Geometry check sheet. Reference: the model listing, model coordinates, mm. Face numbers are marked on the shaded views. A direction names the side the tool comes from. Coordinates: 2 decimals unless noted, no trailing zeros. Loops run counter-clockwise (first coordinate to the right, second up) from the corner with the lowest first, then second, coordinate; pieces in that order, holes last. Notation, with made-up numbers: (82.5, 26.25) -> (120.5, 26.25) arc R11 ccw to (120.5, 37.25) -> close; hole circle Ø3 at (45.5, 13). An arc over 180 degrees is marked (long way). Answer as a JSON object with one key per item and string values.
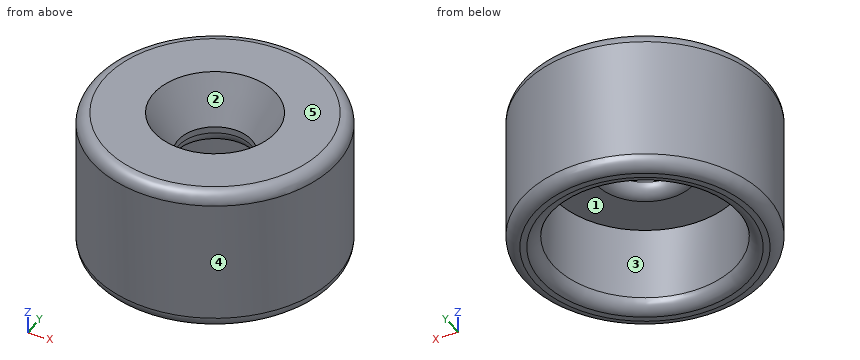
from build123d import *

# Parameters (mm, degrees)
SKETCH1_R           = 5
SKETCH1_R_2         = 1.5
BOSS_EXTRUDE1_DEPTH = 6
SKETCH2_R           = 3.75
CUT_EXTRUDE1_DEPTH  = 3.5
FILLET1_R           = 0.5
CHAMFER1_SIZE       = 1
CHAMFER1_SIZE2      = 1.732050808


with BuildPart() as part:
    # Sketch1 → Boss-Extrude1 (new body)
    with BuildSketch(Plane.XY):
        Circle(SKETCH1_R)
        Circle(SKETCH1_R_2, mode=Mode.SUBTRACT)
    extrude(amount=BOSS_EXTRUDE1_DEPTH)

    # Sketch2 → Cut-Extrude1 (cut)
    with BuildSketch(Plane.XY):
        Circle(SKETCH2_R)
    extrude(amount=CUT_EXTRUDE1_DEPTH, mode=Mode.SUBTRACT)

    # Fillet1
    fillet1_edges = [part.edges().sort_by_distance(p)[0] for p in [
        (-1.5, 0, 3.5),
        (-3.75, 0, 0),
        (-5, 0, 0),
        (-5, 0, 6),
    ]]
    fillet(fillet1_edges, radius=FILLET1_R)

    # Chamfer1
    chamfer1_edges = [part.edges().sort_by_distance(p)[0] for p in [
        (-1.5, 0, 6),
    ]]
    chamfer1_side = [part.faces().sort_by_distance(p)[0] for p in [
        (-4.372720779, 0, 6),
    ]]
    chamfer(chamfer1_edges, length=CHAMFER1_SIZE, length2=CHAMFER1_SIZE2, reference=chamfer1_side[0])


solid = part.part
1. Tool access check on the marked faces 1 and 2. Record the directions out of +Z, -Z, +X, -X, +Y, -Y that give a thin tool (end or side, any length) a straight path to the whole face; none if there is none.
Evaluation:
{"face 1": "-Z", "face 2": "+Z"}
2. Section check D-D, the plane z = 5.1. Record the boundary of the cut face in (x, y).
Evaluation:
{"outline": "circle Ø10 at (0, 0); hole circle Ø3.96 at (0, 0)"}
3. Thickness scan on probe 1 along Y at (x, z) = (0, 2.8); probe 2 along Y at (x, z) = (0, 4.1); probe 3 along X at (y, z) = (0.5, 5.4). Record the ranges inside material, lowest first. Write a range as from..to.
Evaluation:
{"probe 1": "y = -5..-3.75, 3.75..5", "probe 2": "y = -5..-1.5, 1.5..5", "probe 3": "x = -4.97..-2.09, 2.09..4.97"}
4. Section check A-A, the plane y = 0. Record the boundary of the cut face in (x, z).
Evaluation:
{"outline": "(-5, 0.5) arc R0.5 ccw to (-4.5, 0) -> (-4.25, 0) arc R0.5 ccw to (-3.75, 0.5) -> (-3.75, 3.5) -> (-2, 3.5) arc R0.5 ccw to (-1.5, 4) -> (-1.5, 4.27) -> (-2.5, 6) -> (-4.5, 6) arc R0.5 ccw to (-5, 5.5) -> close; (1.5, 4) arc R0.5 ccw to (2, 3.5) -> (3.75, 3.5) -> (3.75, 0.5) arc R0.5 ccw to (4.25, 0) -> (4.5, 0) arc R0.5 ccw to (5, 0.5) -> (5, 5.5) arc R0.5 ccw to (4.5, 6) -> (2.5, 6) -> (1.5, 4.27) -> close"}
5. Section check C-C, the plane z = 3. Record the boundary of the cut face in (x, y).
Evaluation:
{"outline": "circle Ø10 at (0, 0); hole circle Ø7.5 at (0, 0)"}
6. Depth check by flat-ended pin: P1, Ø6, axis at x = 0, y = -1, coming from the -Z side; P2, Ø1, axis at x = 2.5, z = 4.5, coming from the +Y side; P3, Ø2, axis at y = 2.5, z = 3, coming from the +X side; P4, Ø2.5, axis at x = 0, y = 0, coming from the +Z side. Enter the tip coordinate at first touch or a pass-through.
Evaluation:
{"P1": "stops at z = 0.07", "P2": "stops at y = 4.58", "P3": "stops at x = 4.77", "P4": "passes through"}
7. Mould release check, pull along Y, two halves, no side actions. Record for the marked faces 3, 4 and 5: released by +Y, released by -Y, zero draft, split by the parting line, or undercut.
Evaluation:
{"face 3": "undercut", "face 4": "split by the parting line", "face 5": "zero draft"}
